Read the model definition and answer for the solid it produces. Units are mm, in the model's axes. Coordinates: 2 decimals unless noted, no trailing zeros. Write each loop counter-clockwise with the first axis right and the second up, starting at its lowest first coordinate (ties: lowest second). Pieces come first, ordered by that corner, then holes.
1) The part is cut by section A-A (z = 0.5). Determine the outline of the cut face in (x, y).
2) Find the intervals of material crossed by line 1 (X direction, y = 2.8, z = 0.8); line 2 (X direction, y = 2.45, z = 0.55); line 3 (X direction, y = 2.6, z = 1.6), in increasing order.
3) Determine the mould class of faces 1 (the face through (68, 2, 3)), 2 (the face through (-2, 2, 1)), 3 (the face through (141, 2, 1)) for opening direction X: +X half, -X half, draft (parallel to the pull), parting line (faces both ways), or undercut.
from build123d import *

# Parameters (mm, degrees)
EXTRUDE_1_DEPTH = 3


with BuildPart() as part:
    # 草图1 → 凸台-拉伸1 (new body)
    with BuildSketch(Plane.XY):
        with BuildLine():
            Line((0, 0), (139, 0))
            ThreePointArc((139, 0), (141, 2), (139, 4))
            Line((139, 4), (0, 4))
            ThreePointArc((0, 4), (-2, 2), (0, 0))
        make_face()
    extrude(amount=EXTRUDE_1_DEPTH)

    # 草图2 → 切除-旋转1 (revolve, cut)
    with BuildSketch(Plane(origin=(0, 2, 0), x_dir=(-1, 0, 0), z_dir=(0, -1, 0))):
        with BuildLine():
            Line((0, -0.5), (0, 0))
            Line((0, 0), (0, 0.5))
            ThreePointArc((0, 0.5), (-1, -0.5), (0, -1.5))
            Line((0, -1.5), (0, -0.5))
        make_face()
    revolve(axis=Axis((0, 2, 0), (0, 0, -1)), mode=Mode.SUBTRACT)

    # 草图4 → 切除-旋转3 (revolve, cut)
    with BuildSketch(Plane(origin=(0, 2, 0), x_dir=(-1, 0, 0), z_dir=(0, -1, 0))):
        with BuildLine():
            Line((-139, -0.5), (-139, 0))
            Line((-139, 0), (-139, 0.5))
            ThreePointArc((-139, 0.5), (-140, -0.5), (-139, -1.5))
            Line((-139, -1.5), (-139, -0.5))
        make_face()
    revolve(axis=Axis((139, 2, 1.5), (0, 0, -1)), mode=Mode.SUBTRACT)


solid = part.part
Reported:
1. outline: (0, 0) - (139, 0) arc R2 ccw to (139, 4) - (0, 4) arc R2 ccw to start; hole circle Ø2 at (0, 2); hole circle Ø2 at (139, 2)
2. line 1: x = -1.83 to -0.52, 0.52 to 138.48, 139.52 to 140.83
2. line 2: x = -1.95 to -0.89, 0.89 to 138.11, 139.89 to 140.95
2. line 3: x = -1.91 to 140.91
3. face 1: draft
3. face 2: -X half
3. face 3: +X half
